Geometry check sheet. Reference: the model listing, model coordinates, mm. A direction names the side the tool comes from. Round coordinates to 2 decimals unless told otherwise and drop trailing zeros. Loops run counter-clockwise (first coordinate to the right, second up) from the corner with the lowest first, then second, coordinate; pieces in that order, holes last.
Solid Edge part; units mm, degrees
sketch "Sketch1" plane through (0, 0, 0) normal (0, 0, 1) x (1, 0, 0)
  line L0 (-86, -15) -> (-2.9372, -24.8269)
  line L1 (-86, 15) -> (-2.9372, 24.8269)
  line L2 (-110, 15) -> (-86, 15)
  line L3 (-110, 0) -> (-110, 15)
  line L4 (-110, 0) -> (-110, -15)
  line L5 (-110, -15) -> (-86, -15)
  arc A0 (-2.9372, 24.8269) -> (-2.9372, -24.8269) centre (0, 0) cw
extrude "Protrusion1" add sketch "Sketch1" along normal mid plane 10
sketch "Sketch2" plane through (-42.5, 0, 5) normal (0, 0, 1) x (0.9930744, -0.117487, 0)
  circle A0 centre (42.2057, 4.9932) radius 25
extrude "ExtrudedProtrusion_2" add sketch "Sketch2" along normal mid plane 50
sketch "Sketch3" plane through (-42.5, 0, 5) normal (0, 0, 1) x (0.9930744, -0.117487, 0)
  circle A0 centre (42.2057, 4.9932) radius 15
extrude "Cutout1" cut sketch "Sketch3" along normal through all and the other way through all
sketch "Sketch4" plane through (-98, -15, 0) normal (0, -1, 0) x (1, 0, 0)
  line L0 (12, 20) -> (12, -5)
  arc A0 (-12, 20) -> (12, 20) centre (0, 20) cw
  line L1 (-12, -5) -> (-12, 20)
extrude "ExtrudedProtrusion_3" add sketch "Sketch4" against normal blind 9 material side at (-85.95, -15, 7.5)
sketch "Sketch5" plane through (-98, 15, 0) normal (0, 1, 0) x (-1, 0, 0)
  line L0 (12, 20) -> (12, -5)
  arc A0 (-12, 20) -> (12, 20) centre (0, 20) cw
  line L1 (-12, -5) -> (-12, 20)
extrude "ExtrudedProtrusion_4" add sketch "Sketch5" against normal blind 9 material side at (-110.05, 15, 7.5)
sketch "Sketch6" plane through (-98, -15, 0) normal (0, -1, 0) x (1, 0, 0)
  circle A0 centre (0, 20) radius 6
extrude "Cutout2" cut sketch "Sketch6" against normal through all
1) Mould release check, pull along X, two halves, no side actions. Record for faces 1 (the face through (-57, 0, -5)), 2 (the face through (-45.05, -19.845, -0.07)), 3 (the face through (-98, 11, 32)): +X half, -X half, draft (parallel to the pull), parting line (faces both ways), or undercut.
Report:
face 1: draft
face 2: -X half
face 3: undercut
2) Sectioned sample at C-C, the plane x = 0. Record the cut outline in (y, z), then the cut area to 3 significant figures.
Report:
outline: (-25, -20) - (-15, -20) - (-15, 30) - (-25, 30) - close; (15, -20) - (25, -20) - (25, 30) - (15, 30) - close
area: 1,000 mm2
3) Sectioned sample at D-D, the plane y = 0. Record the cut outline in (x, z).
Report:
outline: (-110, -5) - (-25, -5) - (-25, -20) - (-15, -20) - (-15, 30) - (-25, 30) - (-25, 5) - (-110, 5) - close; (15, -20) - (25, -20) - (25, -5) - (25, 30) - (15, 30) - close
4) Access from +Z, -Z, +X, -X, +Y, -Y to the whole of each face (thin tool, end or side, straight path). Record for faces 4 (the face through (-98, 15, 10)), 5 (the face through (-86, 11, 12)), 6 (the face through (-57, 0, 5)), 7 (the face through (11, -11, 30)).
Report:
face 4: +Z, -Z, -X, +Y
face 5: +Z, +Y, -Y
face 6: +Z
face 7: +Z, +X, +Y, -Y
5) Scan lines: line 1 along X through (y, z) = (13, 29); line 2 along X through (y, z) = (8.5, 11); line 3 along X through (y, z) = (-9.5, 23). Record each from-to range of solid material in increasing order.
Report:
line 1: x = -105.94 to -90.06, -21.35 to -7.48, 7.48 to 21.35
line 2: x = -110 to -86, -23.51 to -12.36, 12.36 to 23.51
line 3: x = -109.62 to -103.2, -92.8 to -86.38, -23.12 to -11.61, 11.61 to 23.12
6) Gauge pin test, flat ends, axial feed: pin 1 (1 mm diameter, centred on x = -27, z = -9.5, fed in from +Y); pin 2 (7 mm diameter, centred on x = -94, z = 15.5, fed in from -Y); pin 3 (12 mm diameter, centred on x = -100.5, z = 13.5, fed in from +Y); pin 4 (12 mm diameter, centred on y = -15.5, z = -11.5, fed in from +X). Record the tip position at first contact, or that the pin passes through.
Report:
pin 1: passes through
pin 2: stops at y = -15
pin 3: stops at y = 15
pin 4: stops at x = 23.12
7) Sectioned sample at B-B, the plane y = -13.5. Record the cut outline in (x, z), then the cut area to 3 significant figures.
Report:
outline: (-110, -5) - (-21.04, -5) - (-21.04, -20) - (-6.54, -20) - (-6.54, 30) - (-21.04, 30) - (-21.04, 5) - (-86, 5) - (-86, 20) arc R12 ccw to (-110, 20) - close; (6.54, -20) - (21.04, -20) - (21.04, -5) - (21.04, 30) - (6.54, 30) - close; hole circle Ø12 at (-98, 20)
area: 2,810 mm2
8) Sectioned sample at A-A, the plane x = -98. Record the cut outline in (y, z).
Report:
outline: (-15, -5) - (15, -5) - (15, 14) - (6, 14) - (6, 5) - (-6, 5) - (-6, 14) - (-15, 14) - close; (-15, 26) - (-6, 26) - (-6, 32) - (-15, 32) - close; (6, 26) - (15, 26) - (15, 32) - (6, 32) - close
